Could you check a few things on this model? Use its own coordinates, in mm. Give positions to 0.01 mm unless a question says otherwise; leave off trailing zeros. Loops run counter-clockwise (first coordinate to the right, second up) from the corner with the lowest first, then second, coordinate; pieces in that order, holes last. Notation, with made-up numbers: (-22, -3) -> (-16, -3) arc R30 ccw to (-16, 30) -> close; hole circle Ø4 at (67, -22). An arc over 180 degrees is marked (long way). Write item = value, one per line. Start each with the question number.
1) I'm going to push flat-ended pins straight in: pin 1 Ø1 at (y, z) = (21.5, -63) entering from -X; pin 2 Ø9 at (x, z) = (-18, -192.5) entering from +Y; pin 3 Ø2 at (y, z) = (25, -173.5) entering from +X (3 decimals); pin 4 Ø6 at (x, y) = (-18, 15) entering from +Z. Where does each tip first touch, or does it pass through?
2) I want a section at C-C (y = 16). List the corners of the cut face in (x, z) for me, and give its area (3 significant figures).
3) I want a section at A-A (x = -7). List the corners of the cut face in (y, z) for me, and give its area (3 significant figures).
4) I need wall thicknesses on probe 1 along Y at (x, z) = (-11.25, -121); probe 2 along X at (y, z) = (20.5, -172); probe 3 along X at (y, z) = (26.5, -279.5) (3 decimals). Which ranges of each line are inside material? Lowest first, please. Write a range as from..to.
from build123d import *

# Parameters (mm, degrees)
EXTRUDE_THIN1_DEPTH = 317.5
FILLET1_R           = 1.27


with BuildPart() as part:
    # Sketch1 → Extrude-Thin1 (new body)
    with BuildSketch(Plane.XY):
        Polygon((0, 0), (-12.7, 0), (-12.7, 22.225), (-22.225, 22.225), (-22.225, 28.575), (-12.7, 30.1625), (-12.7, 31.75), (0, 31.75), (0, 30.48), (-11.43, 30.48), (-11.43, 29.086648598), (-20.955, 27.499148598), (-20.955, 23.495), (-11.43, 23.495), (-11.43, 1.27), (0, 1.27), align=None)
    extrude(amount=-EXTRUDE_THIN1_DEPTH)

    # Fillet1
    fillet1_edges = [part.edges().sort_by_distance(p)[0] for p in [
        (-11.43, 29.086648598, -158.75),
        (-11.43, 23.495, -158.75),
        (-12.7, 0, -158.75),
        (-22.225, 22.225, -158.75),
        (-22.225, 28.575, -158.75),
        (-12.7, 31.75, -158.75),
    ]]
    fillet(fillet1_edges, radius=FILLET1_R)


solid = part.part
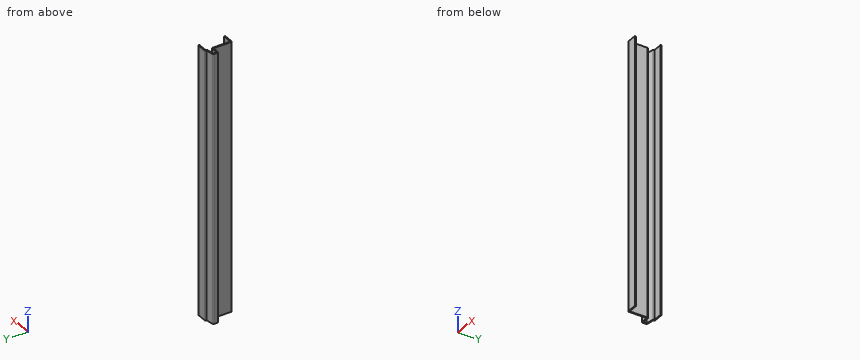
Answer list:
q1.pin_1 = -12.7
q1.pin_2 = 30.03
q1.pin_3 = -20.955
q1.pin_4 = through
q2.outline = (-12.7, -317.5) -> (-11.43, -317.5) -> (-11.43, 0) -> (-12.7, 0) -> close
q2.area = 403 mm^2
q3.outline = (0, -317.5) -> (1.27, -317.5) -> (1.27, 0) -> (0, 0) -> close; (30.48, -317.5) -> (31.75, -317.5) -> (31.75, 0) -> (30.48, 0) -> close
q3.area = 806 mm^2
q4.probe_1 = 0..1.27, 30.48..31.75
q4.probe_2 = -12.7..-11.43
q4.probe_3 = -22.225..-20.955
